Check sheet for the drawn part. Datum: minimum x, y, z corner. Units: mm. A direction names the side the tool comes from. Round coordinates to 2 decimals unless told otherwise and drop trailing zeros. Order: outer loops, then holes, each group sorted by start corner. A loop starts at its lowest first (then second) coordinate and runs counter-clockwise, first axis right, second up. Notation, with made-up numbers: M 1.25,52 L 57.25,52 A18 cw 57.25,70 Z; hole C -8.5,72.5 d8. An arc over 180 degrees is marked long. Answer as a JSON object with one key per item and string values. Group by question number.
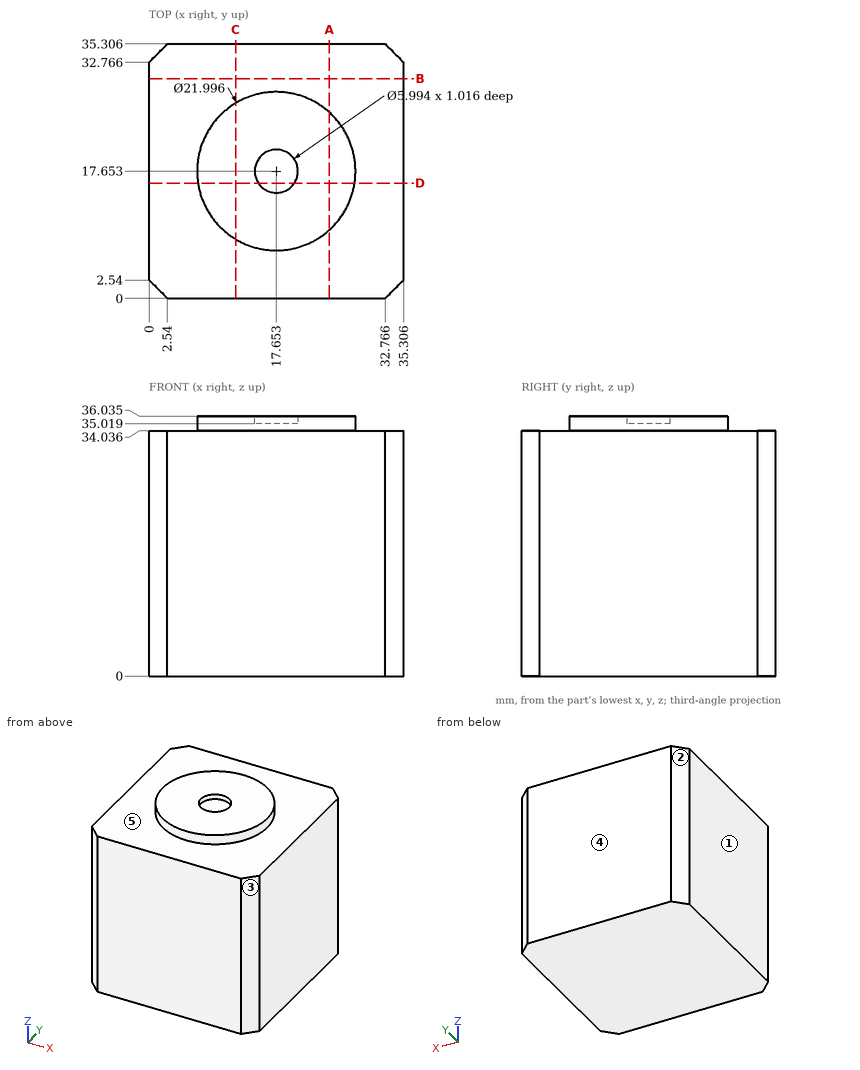
1) Set-up check for the marked faces 4 and 5: record each of +Z, -Z, +X, -X, +Y, -Y from which the full face is reachable in a straight line by a thin tool's end or side.
2) Thickness scan on line 1 along Z through (x, y) = (30.5, 34.5); line 2 along Z through (x, y) = (17, 17); line 3 along Y through (x, z) = (33.5, 28.5) (1 decimal). Record the ranges inside material, lowest first. Write a range as [from, to].
3) Release check for a two-part mould opening along Y. For the marked faces 1, 2 and 3 record: +Y half, -Y half, draft (parallel to the pull), parting line (faces both ways), or undercut.
4) Go/stop test with a flat-tipped pin: P1, Ø2, axis at y = 21.5, z = 29, coming from the -X side. Record where the tip stops, or that it passes through.
5) Sectioned sample at D-D (y = 16). Record the boundary of the cut face in (x, z) (1 decimal), then the cut area to 3 significant figures.
6) Sectioned sample at A-A (x = 25). Record the boundary of the cut face in (y, z) (1 decimal).
7) Sectioned sample at C-C (x = 12). Record the boundary of the cut face in (y, z) (1 decimal).
8) Sectioned sample at B-B (y = 30.5). Record the boundary of the cut face in (x, z), then the cut area to 3 significant figures.
Final values:
{
 "1": {"face 4": "+Z, -Z, +X, -X, +Y", "face 5": "+Z"},
 "2": {"line 1": "z = [0, 34.04]", "line 2": "z = [0, 35.02]", "line 3": "y = [0.7, 34.6]"},
 "3": {"face 1": "draft", "face 2": "+Y half", "face 3": "-Y half"},
 "4": {"P1": "stops at x = 0"},
 "5": {"outline": "M 0,0 L 35.3,0 L 35.3,34 L 28.5,34 L 28.5,36 L 20.2,36 L 20.2,35 L 15.2,35 L 15.2,36 L 6.8,36 L 6.8,34 L 0,34 Z", "area": "1,240 mm^2"},
 "6": {"outline": "M 0,0 L 35.3,0 L 35.3,34 L 25.8,34 L 25.8,36 L 9.5,36 L 9.5,34 L 0,34 Z"},
 "7": {"outline": "M 0,0 L 35.3,0 L 35.3,34 L 27.1,34 L 27.1,36 L 8.2,36 L 8.2,34 L 0,34 Z"},
 "8": {"outline": "M 0,0 L 35.31,0 L 35.31,34.04 L 0,34.04 Z", "area": "1,200 mm^2"}
}
